Design review of the part shown in the three views and the two pictorial views. Dimensions are in mm from the part's minimum x, y and z. A direction names the side the tool comes from. Give positions to 0.01 mm unless a question says otherwise; leave off trailing zeros. Order: outer loops, then holes, each group sorted by start corner. A loop starts at its lowest first (then second) coordinate and runs counter-clockwise, first axis right, second up.
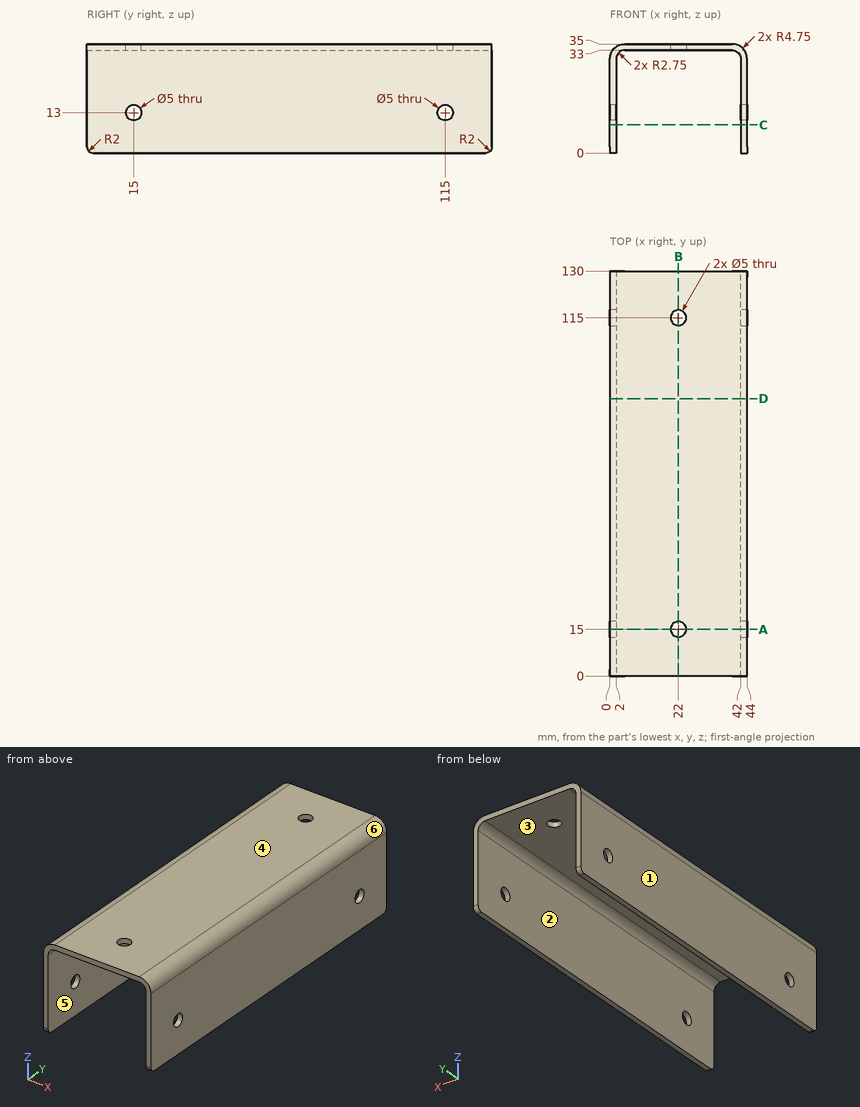
Item 1: Take a section at D-D (y = 89). Give the boundary of the cut face in (x, z).
Values found:
outline: (0, 0) - (2, 0) - (2, 30.25) arc R2.75 cw to (4.75, 33) - (39.25, 33) arc R2.75 cw to (42, 30.25) - (42, 0) - (44, 0) - (44, 30.25) arc R4.75 ccw to (39.25, 35) - (4.75, 35) arc R4.75 ccw to (0, 30.25) - close
Item 2: Take a section at A-A (y = 15). Give the boundary of the cut face in (x, z), and give its area (3 significant figures).
Values found:
outline: (0, 0) - (2, 0) - (2, 10.5) - (0, 10.5) - close; (0, 15.5) - (2, 15.5) - (2, 30.25) arc R2.75 cw to (4.75, 33) - (19.5, 33) - (19.5, 35) - (4.75, 35) arc R4.75 ccw to (0, 30.25) - close; (24.5, 33) - (39.25, 33) arc R2.75 cw to (42, 30.25) - (42, 15.5) - (44, 15.5) - (44, 30.25) arc R4.75 ccw to (39.25, 35) - (24.5, 35) - close; (42, 0) - (44, 0) - (44, 10.5) - (42, 10.5) - close
area: 184 mm2
Item 3: For the marked faces 5 and 6, list the 3-axis set-ups (+Z, -Z, +X, -X, +Y, -Y) from which the entire face can be reached by the end or side of a thin tool; tool diameter is ignored.
Values found:
face 5: -Z, +Y, -Y
face 6: +Z, +X, +Y, -Y
Item 4: Take a section at C-C (z = 9). Give the boundary of the cut face in (x, y), and give its area (3 significant figures).
Values found:
outline: (0, 0) - (2, 0) - (2, 130) - (0, 130) - close; (42, 0) - (44, 0) - (44, 130) - (42, 130) - close
area: 520 mm2
Item 5: Take a section at B-B (x = 22). Give the boundary of the cut face in (y, z), and give its area (3 significant figures).
Values found:
outline: (0, 33) - (12.5, 33) - (12.5, 35) - (0, 35) - close; (17.5, 33) - (112.5, 33) - (112.5, 35) - (17.5, 35) - close; (117.5, 33) - (130, 33) - (130, 35) - (117.5, 35) - close
area: 240 mm2
Item 6: Draft analysis for pull direction X (two halves, no side actions). For the marked faces 1, 2, 3 and 4, state which applies: released by +X, released by -X, zero draft, split by the parting line, or undercut.
Values found:
face 1: released by -X
face 2: undercut
face 3: undercut
face 4: zero draft
Item 7: Clearance check with a flat-ended pin moving along its axis: pin 1 Ø10.5 at (x, y) = (19, 40.5) entering from -Z. State where the tip first meets the part, or that it passes through.
Values found:
pin 1: stops at z = 33
Item 8: For line 1 (X direction, y = 87, z = 3); line 2 (Z direction, x = 16.5, y = 19); line 3 (Z direction, x = 1.25, y = 15), list the stretches that pass through material, from the lowest coordinate up.
Values found:
line 1: x = 0 to 2, 42 to 44
line 2: z = 33 to 35
line 3: z = 0 to 10.5, 15.5 to 33.46
